```python
from build123d import *

# Parameters (mm, degrees)
EXTRUDE_1_DEPTH     = 3
SKETCH_2_R          = 3
CUT_EXTRUDE_1_DEPTH = 146.275600154


with BuildPart() as part:
    # Эскиз1 → Бобышка-Вытянуть1 (new body)
    with BuildSketch(Plane(origin=(0, 0, 0), x_dir=(0, 0, -1), z_dir=(1, 0, 0))):
        Polygon((0, 65), (0, 25), (3, 25), (3, 3), (32, 3), (32, 0), (82, 0), (82, 3), (111, 3), (111, 25), (114, 25), (114, 65), (111, 65), (111, 87), (82, 87), (82, 90), (32, 90), (32, 87), (3, 87), (3, 65), align=None)
    extrude(amount=EXTRUDE_1_DEPTH)

    # Эскиз2 → Вырез-Вытянуть1 (cut, through all)
    with BuildSketch(Plane(origin=(3, 0, 0), x_dir=(0, 0, -1), z_dir=(1, 0, 0))):
        with Locations((32, 45)):
            Circle(SKETCH_2_R)
        with Locations((35.349364905, 57.5)):
            Circle(SKETCH_2_R)
        with Locations((44.5, 66.650635095)):
            Circle(SKETCH_2_R)
        with Locations((57, 70)):
            Circle(SKETCH_2_R)
        with Locations((69.5, 66.650635095)):
            Circle(SKETCH_2_R)
        with Locations((78.650635095, 57.5)):
            Circle(SKETCH_2_R)
        with Locations((82, 45)):
            Circle(SKETCH_2_R)
        with Locations((78.650635095, 32.5)):
            Circle(SKETCH_2_R)
        with Locations((69.5, 23.349364905)):
            Circle(SKETCH_2_R)
        with Locations((57, 20)):
            Circle(SKETCH_2_R)
        with Locations((44.5, 23.349364905)):
            Circle(SKETCH_2_R)
        with Locations((35.349364905, 32.5)):
            Circle(SKETCH_2_R)
    extrude(amount=-CUT_EXTRUDE_1_DEPTH, mode=Mode.SUBTRACT)


solid = part.part
```
CAD build for the part. Positions are in the model's coordinates, mm. A direction names the side the tool comes from. Round coordinates to 2 decimals unless told otherwise and drop trailing zeros. Order: outer loops, then holes, each group sorted by start corner. A loop starts at its lowest first (then second) coordinate and runs counter-clockwise, first axis right, second up.
Item 1: Tool access for faces 5 (the face through (1, 76, -111)), 6 (the face through (1, 14, -111)), 7 (the face through (1, 2, -32)): list every direction of +Z, -Z, +X, -X, +Y, -Y with a clear straight run to the whole face (end or side of a thin tool).
Item 2: Mould opens along Y. For faces 1 (the face through (1, 45, -114)), 2 (the face through (2, 20, -54)), 3 (the face through (1, 0, -57)), 4 (the face through (1.521, 58.401, -81.512)) say: pulls with the +Y half, pulls with the -Y half, needs draft (parallel to the pull), parting line crosses it, or undercut.
Item 3: Saw through at C-C on x = 2.35. State how many separate pieces and enclosed holes the cut face has, then the cut area to 3 significant figures.
Item 4: Saw through at A-A on y = 57.5. Write the cut outline in (x, z).
Item 5: Saw through at B-B on z = -69.5. Write the cut outline in (x, y), then the cut area to 3 significant figures.
Item 6: Saw through at D-D on z = -96. Write the cut outline in (x, y).
Item 7: Probe line 1 along Z through (x, y) = (1.05, 55); line 2 along Y through (x, z) = (1, -76); line 3 along Z through (x, y) = (2.6, 26). List the from-to ranges inside material, lowest first.
Item 8: Pin check, flat tips, straight feed: pin 1 (5.5 mm diameter, centred on y = 45, z = -82, fed in from +X); pin 2 (1.5 mm diameter, centred on x = 1.5, z = -17.5, fed in from -Y). Stop position of each tip, or through.
Reported:
1. face 5: -Z, +X, -X, +Y
1. face 6: -Z, +X, -X, -Y
1. face 7: +Z, +X, -X, -Y
2. face 1: needs draft
2. face 2: undercut
2. face 3: pulls with the -Y half
2. face 4: undercut
3. separate pieces: 1
3. enclosed holes: 12
3. area: 9,270 mm2
4. outline: (0, -114) - (3, -114) - (3, -81.65) - (0, -81.65) - close; (0, -75.65) - (3, -75.65) - (3, -38.35) - (0, -38.35) - close; (0, -32.35) - (3, -32.35) - (3, 0) - (0, 0) - close
5. outline: (0, 0) - (3, 0) - (3, 20.35) - (0, 20.35) - close; (0, 26.35) - (3, 26.35) - (3, 63.65) - (0, 63.65) - close; (0, 69.65) - (3, 69.65) - (3, 90) - (0, 90) - close
5. area: 234 mm2
6. outline: (0, 3) - (3, 3) - (3, 87) - (0, 87) - close
7. line 1: z = -114 to -80.31, -76.99 to -37.01, -33.69 to 0
7. line 2: y = 0 to 31.09, 33.91 to 56.09, 58.91 to 90
7. line 3: z = -114 to -70.91, -68.09 to -45.91, -43.09 to 0
8. pin 1: passes through
8. pin 2: stops at y = 3
